```python
from build123d import *

# Parameters (mm, degrees)
F0_W     = 16.9
F0_H     = 14.5
F0_W_2   = 16
F0_H_2   = 18
F0_W_3   = 2.4
F0_H_3   = 10
F1_DEPTH = 2.4


with BuildPart() as f1:
    # F0 (on Top) → F1 (new body)
    with BuildSketch(Plane.XY):
        Polygon((32.5, -20), (32.5, 20), (25, 20), (25, 22.4), (15, 22.4), (15, 20), (-15, 20), (-15, 22.4), (-25, 22.4), (-25, 20), (-32.5, 20), (-32.5, -20), (-25, -20), (-25, -22.4), (-15, -22.4), (-15, -20), (7.5, -20), (15, -20), (15, -22.4), (25, -22.4), (25, -20), align=None)
        with Locations((-17.75, -6.65)):
            Rectangle(F0_W, F0_H, mode=Mode.SUBTRACT)
        with Locations((0.95, -4.9)):
            Rectangle(F0_W_2, F0_H_2, mode=Mode.SUBTRACT)
        with Locations((19.05, -4.9)):
            Rectangle(F0_W_2, F0_H_2, mode=Mode.SUBTRACT)
        with Locations((-29.8, 0)):
            Rectangle(F0_W_3, F0_H_3, mode=Mode.SUBTRACT)
        with Locations((29.8, 0)):
            Rectangle(F0_W_3, F0_H_3, mode=Mode.SUBTRACT)
    extrude(amount=F1_DEPTH)


solid = f1.part
```
Here's how the part is built. I have some questions about the finished solid (model axes, mm). A direction names the side the tool comes from. Give positions to 0.01 mm unless a question says otherwise; leave off trailing zeros. Order: outer loops, then holes, each group sorted by start corner. A loop starts at its lowest first (then second) coordinate and runs counter-clockwise, first axis right, second up. Notation, with made-up numbers: (14.5, 26.25) - (69.5, 26.25) arc R30 cw to (69.5, 55.25) - close; hole circle Ø9 at (55.5, -31.5). An arc over 180 degrees is marked (long way). Answer as a JSON object with one key per item and string values. Group by question number.
Item 1: If we section it at A-A on y = -8.5: Please give me the cut outline in (x, z), and give its area (3 significant figures).
Item 2: If we section it at B-B on x = -22: Please give me the cut outline in (y, z), and give its area (3 significant figures).
Item 3: If we section it at C-C on y = 3: Please give me the cut outline in (x, z).
Item 4: Which directions (+Z, -Z, +X, -X, +Y, -Y) give clear straight access to the entire face, cutting with the end or side of a thin tool? Please do faces 4 (the flat face through (-29, -20, 1)), 5 (the flat face through (-15, 21, 1)), 6 (the flat face through (-30, 5, 1)).
Item 5: If we mould it in two halves opening along Y, with no side actions, what happens to faces 1 (the flat face through (-30, -5, 1)), 2 (the flat face through (0, 5, 0)), 3 (the flat face through (-29, 20, 1))? For each: pulls with the +Y half, pulls with the -Y half, needs draft (parallel to the pull), parting line crosses it, or undercut.
Item 6: If we section it at D-D on z = 0.7: Give the number of separate pieces and of enclosed holes in the cut face, and give its area (3 significant figures).
Item 7: For P1, Ø0.7, axis at y = -21, z = 1, coming from the +X side; P2, Ø1.2, axis at x = -29.5, z = 0.5, coming from the +Y side; P3, Ø1.2, axis at x = 28, z = 1, coming from the -Y side, each with a flat end and sliding along its axis, tell me the tip position at first contact or that it passes through.
Item 8: Please list where these lines run through material, in increasing order: probe 1 along X at (y, z) = (4, 1.95); probe 2 along X at (y, z) = (-11, 1.05); probe 3 along X at (y, z) = (-4, 1.4).
Result set:
{
 "1": {"outline": "(-32.5, 0) - (-26.2, 0) - (-26.2, 2.4) - (-32.5, 2.4) - close; (-9.3, 0) - (-7.05, 0) - (-7.05, 2.4) - (-9.3, 2.4) - close; (8.95, 0) - (11.05, 0) - (11.05, 2.4) - (8.95, 2.4) - close; (27.05, 0) - (32.5, 0) - (32.5, 2.4) - (27.05, 2.4) - close", "area": "38.6 mm²"},
 "2": {"outline": "(-22.4, 0) - (-13.9, 0) - (-13.9, 2.4) - (-22.4, 2.4) - close; (0.6, 0) - (22.4, 0) - (22.4, 2.4) - (0.6, 2.4) - close", "area": "72.7 mm²"},
 "3": {"outline": "(-32.5, 0) - (-31, 0) - (-31, 2.4) - (-32.5, 2.4) - close; (-28.6, 0) - (-7.05, 0) - (-7.05, 2.4) - (-28.6, 2.4) - close; (8.95, 0) - (11.05, 0) - (11.05, 2.4) - (8.95, 2.4) - close; (27.05, 0) - (28.6, 0) - (28.6, 2.4) - (27.05, 2.4) - close; (31, 0) - (32.5, 0) - (32.5, 2.4) - (31, 2.4) - close"},
 "4": {"face 4": "+Z, -Z, -X, -Y", "face 5": "+Z, -Z, +Y", "face 6": "+Z, -Z"},
 "5": {"face 1": "undercut", "face 2": "needs draft", "face 3": "pulls with the +Y half"},
 "6": {"separate pieces": "1", "enclosed holes": "5", "area": "1,830 mm²"},
 "7": {"P1": "x = 25", "P2": "y = 20", "P3": "y = -20"},
 "8": {"probe 1": "-32.5 to -31, -28.6 to -7.05, 8.95 to 11.05, 27.05 to 28.6, 31 to 32.5", "probe 2": "-32.5 to -26.2, -9.3 to -7.05, 8.95 to 11.05, 27.05 to 32.5", "probe 3": "-32.5 to -31, -28.6 to -26.2, -9.3 to -7.05, 8.95 to 11.05, 27.05 to 28.6, 31 to 32.5"}
}
